Design review of the part built by this model. Coordinates are the model's own, in mm. Face numbers are marked on the shaded views. Give positions to 0.01 mm unless a question says otherwise; leave off trailing zeros. Order: outer loops, then holes, each group sorted by start corner. A loop starts at its lowest first (then second) coordinate and runs counter-clockwise, first axis right, second up. Notation, with made-up numbers: (37, 74.25) -> (59, 74.25) arc R20 ccw to (59, 101.25) -> close; hole circle Ø6 at (-32, 18). An arc over 180 degrees is marked (long way). One line per item, written item: value.
Autodesk Inventor part; units mm, degrees
ref_plane "YZ Plane" through (0, 0, 0) normal (1, 0, 0) x (0, 1, 0)
ref_plane "XZ Plane" through (0, 0, 0) normal (0, 1, 0) x (-1, 0, 0)
ref_plane "XY Plane" through (0, 0, 0) normal (0, 0, 1) x (1, 0, 0)
sketch "Sketch1" plane through (0, 0, 0) normal (0, 0, 1) x (1, 0, 0)
  line L0 (0, 0) -> (67, 0)
  line L1 (67, 0) -> (67, 5)
  line L2 (67, 5) -> (0, 5)
  line L3 (0, 5) -> (0, 0)
  dimension "d0" = 5
  dimension "d1" = 67
extrude "Extrusion1" add sketch "Sketch1" along normal blind 2
sketch "Sketch2" plane through (0, 0, 2) normal (0, 0, 1) x (1, 0, 0)
  line L0 (0, 0) -> (67, 0)
  line L1 (67, 0) -> (67, 5)
  line L2 (67, 5) -> (0, 5)
  line L3 (0, 5) -> (0, 0)
  line L4 (0, 5) -> (5, 5)
  line L5 (5, 5) -> (5, 0)
  line L6 (5, 0) -> (0, 0)
  line L7 (0, 0) -> (0, 5)
  line L8 (31, 5) -> (36, 5)
  line L9 (36, 5) -> (36, 0)
  line L10 (36, 0) -> (31, 0)
  line L11 (31, 0) -> (31, 5)
  line L12 (67, 5) -> (62, 5)
  line L13 (62, 5) -> (62, 0)
  line L14 (62, 0) -> (67, 0)
  line L15 (67, 0) -> (67, 5)
  dimension "d4" = 5
  dimension "d5" = 5
  dimension "d7" = 26
  dimension "d8" = 26
extrude "Extrusion2" add sketch "Sketch2" along normal blind 2 contours L3 L2 L5 L0 | L11 L2 L9 L0 | L13 L2 L1 L0
sketch "Sketch4" plane through (0, 0, 0) normal (0, 0, -1) x (-1, 0, 0)
  line L0 (0, 0) -> (-67, 0)
  line L1 (0, 5) -> (0, 0)
  line L2 (-67, 5) -> (0, 5)
  line L3 (-67, 0) -> (-67, 5)
  line L4 (-67, 2.5) -> (0, 2.5) construction
  line L5 (-33.5, 5) -> (-33.5, 0) construction
  point P0 (-33.5, 2.5)
hole "Hole1" at (33.5, 2.5, 0) direction (0, 0, 1) diameter 2.013 end through all
properties part number "top_conductor" material "Copper, Alloy"
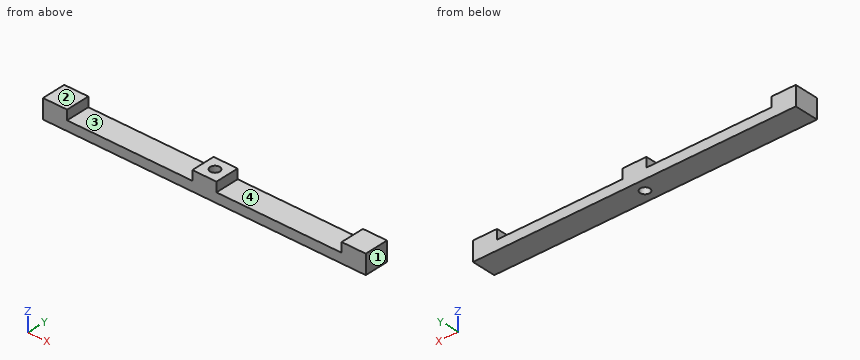
Item 1: Clearance check with a flat-ended pin moving along its axis: P1, Ø3, axis at x = 11.5, y = 3, coming from the +Z side. State where the tip first meets the part, or that it passes through.
Returned:
P1: z = 2
Item 2: Add section A-A on x = 33.5. Give the boundary of the cut face in (y, z), plus the area to 3 significant figures.
Returned:
outline: (0, 0) -> (1.49, 0) -> (1.49, 4) -> (0, 4) -> close; (3.51, 0) -> (5, 0) -> (5, 4) -> (3.51, 4) -> close
area: 11.9 mm²
Item 3: Draft analysis for pull direction X (two halves, no side actions). For the marked faces 1, 2, 3 and 4, state which applies: pulls with the +X half, pulls with the -X half, needs draft (parallel to the pull), parting line crosses it, or undercut.
Returned:
face 1: pulls with the +X half
face 2: needs draft
face 3: undercut
face 4: undercut
Item 4: To check wall thickness, follow line 1 along X through (y, z) = (2.5, 2.3); line 2 along X through (y, z) = (4.8, 2.3); line 3 along Y through (x, z) = (33.5, 1.8). State the ranges of each line that lie inside material, in increasing order. Write a range as from..to.
Returned:
line 1: 0..5, 31..32.49, 34.51..36, 62..67
line 2: 0..5, 31..36, 62..67
line 3: 0..1.49, 3.51..5
Item 5: Add section C-C on z = 2.85. Give the boundary of the cut face in (x, y), plus the area to 3 significant figures.
Returned:
outline: (0, 0) -> (5, 0) -> (5, 5) -> (0, 5) -> close; (31, 0) -> (36, 0) -> (36, 5) -> (31, 5) -> close; (62, 0) -> (67, 0) -> (67, 5) -> (62, 5) -> close; hole circle Ø2.01 at (33.5, 2.5)
area: 71.8 mm²
Item 6: Add section B-B on y = 2.5. Give the boundary of the cut face in (x, z).
Returned:
outline: (0, 0) -> (32.49, 0) -> (32.49, 4) -> (31, 4) -> (31, 2) -> (5, 2) -> (5, 4) -> (0, 4) -> close; (34.51, 0) -> (67, 0) -> (67, 4) -> (62, 4) -> (62, 2) -> (36, 2) -> (36, 4) -> (34.51, 4) -> close
Item 7: Add section D-D on x = 20.5. Give the boundary of the cut face in (y, z).
Returned:
outline: (0, 0) -> (5, 0) -> (5, 2) -> (0, 2) -> close
